from build123d import *

# Parameters (mm, degrees)
SKETCH_1_W          = 65.8
SKETCH_1_H          = 69.8
EXTRUDE_1_DEPTH     = 1.6
SKETCH_2_R          = 1.05
CUT_EXTRUDE_1_DEPTH = 1.6
SKETCH_5_W          = 65.8
SKETCH_5_H          = 69.8
SKETCH_5_W_2        = 62.6
SKETCH_5_H_2        = 66.6
CUT_EXTRUDE_2_DEPTH = 1.6
FILLET_2_R          = 0.4
CHAMFER_1_SIZE      = 0.2


with BuildPart() as part:
    # 草图1 → 凸台-拉伸1 (new body)
    with BuildSketch(Plane(origin=(0, 0, 0), x_dir=(0, 0, -1), z_dir=(1, 0, 0))):
        with Locations((32.9, -34.9)):
            Rectangle(SKETCH_1_W, SKETCH_1_H)
    extrude(amount=EXTRUDE_1_DEPTH)

    # 草图2 → 切除-拉伸1 (cut)
    with BuildSketch(Plane(origin=(1.6, 0, 0), x_dir=(0, 0, -1), z_dir=(1, 0, 0))):
        with Locations((61.2, -4.6)):
            Circle(SKETCH_2_R)
        with Locations((4.4, -4.6)):
            Circle(SKETCH_2_R)
        with Locations((4.4, -65.4)):
            Circle(SKETCH_2_R)
        with Locations((61.2, -65.4)):
            Circle(SKETCH_2_R)
    extrude(amount=-CUT_EXTRUDE_1_DEPTH, mode=Mode.SUBTRACT)

    # 草图5 → 切除-拉伸2 (cut)
    with BuildSketch(Plane.ZY):
        with Locations((-32.9, -34.9)):
            Rectangle(SKETCH_5_W, SKETCH_5_H)
        with Locations((-32.9, -34.9)):
            Rectangle(SKETCH_5_W_2, SKETCH_5_H_2, mode=Mode.SUBTRACT)
    extrude(amount=-CUT_EXTRUDE_2_DEPTH, mode=Mode.SUBTRACT)

    # 圆角2
    fillet_2_edges = [part.edges().sort_by_distance(p)[0] for p in [
        (0.8, -1.6, -1.6),
        (0.8, -68.2, -1.6),
        (0.8, -68.2, -64.2),
        (0.8, -1.6, -64.2),
    ]]
    fillet(fillet_2_edges, radius=FILLET_2_R)

    # 倒角1
    chamfer_1_edges = [part.edges().sort_by_distance(p)[0] for p in [
        (0, -65.4, -60.15),
        (1.6, -65.4, -60.15),
        (0, -65.4, -3.35),
        (1.6, -65.4, -3.35),
        (0, -4.6, -3.35),
        (1.6, -4.6, -3.35),
        (0, -4.6, -60.15),
        (1.6, -4.6, -60.15),
        (0, -34.9, -1.6),
        (1.6, -34.9, -1.6),
        (0, -1.6, -32.9),
        (0, -34.9, -64.2),
        (0, -68.2, -32.9),
        (0, -1.717157288, -64.082842712),
        (0, -68.082842712, -64.082842712),
        (0, -68.082842712, -1.717157288),
        (0, -1.717157288, -1.717157288),
        (1.6, -1.6, -32.9),
        (1.6, -34.9, -64.2),
        (1.6, -68.2, -32.9),
        (1.6, -1.717157288, -64.082842712),
        (1.6, -68.082842712, -64.082842712),
        (1.6, -68.082842712, -1.717157288),
        (1.6, -1.717157288, -1.717157288),
    ]]
    chamfer(chamfer_1_edges, length=CHAMFER_1_SIZE)


solid = part.part
Geometry: final body of the model. Coordinates: model frame, mm. Round coordinates to 2 decimals unless told otherwise and drop trailing zeros. Order: outer loops, then holes, each group sorted by start corner. A loop starts at its lowest first (then second) coordinate and runs counter-clockwise, first axis right, second up. Notation, with made-up numbers: (57.5, 80.25) -> (110.5, 80.25) arc R10 ccw to (110.5, 88.25) -> close; hole circle Ø7 at (22.5, 48). An arc over 180 degrees is marked (long way). Put each result on its own line as item: value. Start each with the question number.
Q1. Line query: probe 1 along Z at (x, y) = (1.1, -4.6); probe 2 along Y at (x, z) = (0.5, -4.4); probe 3 along Y at (x, z) = (0.15, -14). Output: solid intervals per line, ascending.
Q2. Section B-B on z = -4.4. Return the cut outline in (x, y).
Q3. First-contact query: pin 1 (1.9 mm diameter, centred on y = -4.6, z = -4.4, fed in from +X). Flat tip, straight axial feed; report the tip coordinate or a pass-through.
Q4. Pull-direction query (Z, two-part tool) for faces 1 (the flat face through (1.6, -34, -32)), 2 (the cylindrical face through (0.808, -66.332, -61.685)); classes: +Z half, -Z half, draft (parallel to the pull), parting line (faces both ways), or undercut.
Q5. Section A-A on y = -4.6. Return the cut outline in (x, z).
Ans:
1. probe 1: z = -64.2 to -62.25, -60.15 to -5.45, -3.35 to -1.6
1. probe 2: y = -68.2 to -66.45, -64.35 to -5.65, -3.55 to -1.6
1. probe 3: y = -68.15 to -1.65
2. outline: (0, -68) -> (0.2, -68.2) -> (1.4, -68.2) -> (1.6, -68) -> (1.6, -66.65) -> (1.4, -66.45) -> (0.2, -66.45) -> (0, -66.65) -> close; (0, -64.15) -> (0.2, -64.35) -> (1.4, -64.35) -> (1.6, -64.15) -> (1.6, -5.85) -> (1.4, -5.65) -> (0.2, -5.65) -> (0, -5.85) -> close; (0, -3.35) -> (0.2, -3.55) -> (1.4, -3.55) -> (1.6, -3.35) -> (1.6, -1.8) -> (1.4, -1.6) -> (0.2, -1.6) -> (0, -1.8) -> close
3. pin 1: passes through
4. face 1: draft
4. face 2: undercut
5. outline: (0, -64) -> (0.2, -64.2) -> (1.4, -64.2) -> (1.6, -64) -> (1.6, -62.45) -> (1.4, -62.25) -> (0.2, -62.25) -> (0, -62.45) -> close; (0, -59.95) -> (0.2, -60.15) -> (1.4, -60.15) -> (1.6, -59.95) -> (1.6, -5.65) -> (1.4, -5.45) -> (0.2, -5.45) -> (0, -5.65) -> close; (0, -3.15) -> (0.2, -3.35) -> (1.4, -3.35) -> (1.6, -3.15) -> (1.6, -1.8) -> (1.4, -1.6) -> (0.2, -1.6) -> (0, -1.8) -> close
